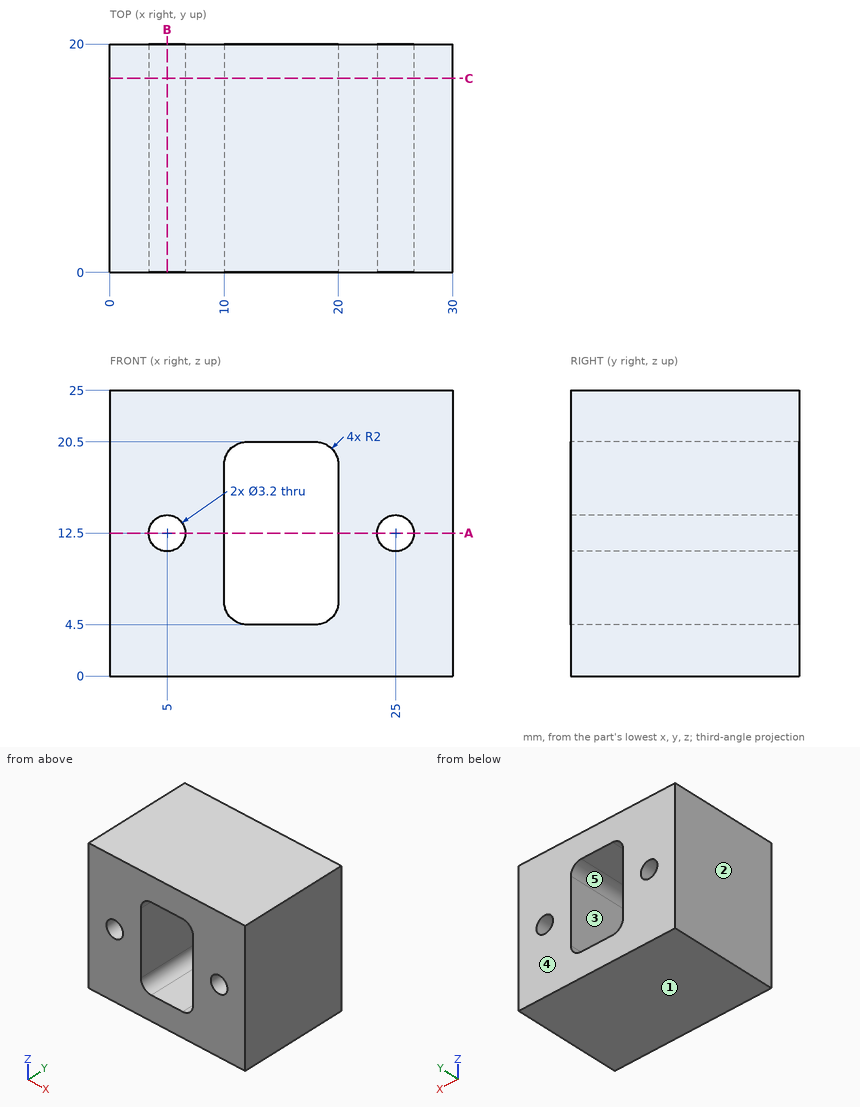
Job drawing, mm, ordinate dimensions from the low corner. One solid piece. A direction names the side the tool comes from. Round coordinates to 2 decimals unless told otherwise and drop trailing zeros. Write each loop counter-clockwise with the first axis right and the second up, starting at its lowest first coordinate (ties: lowest second). Pieces come first, ordered by that corner, then holes. Notation, with made-up numbers: (12.5, 65) -> (25.5, 65) arc R7 cw to (25.5, 69) -> close; hole circle Ø6 at (-39.5, 46). An arc over 180 degrees is marked (long way). Answer as a JSON object with one key per item and string values.
(1) Band-saw the part on C-C, the plane y = 17. List the corners of the cut face in (x, z), then the cut area to 3 significant figures.
Reported:
{"outline": "(0, 0) -> (30, 0) -> (30, 25) -> (0, 25) -> close; hole circle Ø3.2 at (5, 12.5); hole (10, 6.5) arc R2 ccw to (12, 4.5) -> (18, 4.5) arc R2 ccw to (20, 6.5) -> (20, 18.5) arc R2 ccw to (18, 20.5) -> (12, 20.5) arc R2 ccw to (10, 18.5) -> close; hole circle Ø3.2 at (25, 12.5)", "area": "577 mm^2"}
(2) Pin check, flat tips, straight feed: P1, Ø1.9, axis at x = 25, z = 12.5, coming from the +Y side; P2, Ø1, axis at y = 17.5, z = 16, coming from the -X side. Stop position of each tip, or through.
Reported:
{"P1": "passes through", "P2": "stops at x = 0"}
(3) Which spindle directions (+Z, -Z, +X, -X, +Y, -Y) get a long thin tool onto all of the face, cutting with end or side? Do the marked faces 4 and 5. Say none if no direction does.
Reported:
{"face 4": "+Z, -Z, +X, -X, +Y", "face 5": "+Y, -Y"}
(4) Band-saw the part on A-A, the plane z = 12.5. List the corners of the cut face in (x, y).
Reported:
{"outline": "(0, 0) -> (3.4, 0) -> (3.4, 20) -> (0, 20) -> close; (6.6, 0) -> (10, 0) -> (10, 20) -> (6.6, 20) -> close; (20, 0) -> (23.4, 0) -> (23.4, 20) -> (20, 20) -> close; (26.6, 0) -> (30, 0) -> (30, 20) -> (26.6, 20) -> close"}
(5) Probe probe 1 along X at (y, z) = (2.75, 12.5); probe 2 along X at (y, z) = (7.5, 14.5); probe 3 along Z at (x, y) = (13.5, 15.75). List the from-to ranges inside material, lowest first. Write a range as [from, to].
Reported:
{"probe 1": "x = [0, 3.4], [6.6, 10], [20, 23.4], [26.6, 30]", "probe 2": "x = [0, 10], [20, 30]", "probe 3": "z = [0, 4.5], [20.5, 25]"}
(6) Two-plate mould, pull along X, no slides. Class the marked faces 1, 2 and 3: +X half, -X half, draft (parallel to the pull), parting line (faces both ways), or undercut.
Reported:
{"face 1": "draft", "face 2": "-X half", "face 3": "undercut"}
(7) Band-saw the part on B-B, the plane x = 5. List the corners of the cut face in (y, z).
Reported:
{"outline": "(0, 0) -> (20, 0) -> (20, 10.9) -> (0, 10.9) -> close; (0, 14.1) -> (20, 14.1) -> (20, 25) -> (0, 25) -> close"}
